from build123d import *

# Parameters (mm, degrees)
SKETCH1_W             = 9.495809557
SKETCH1_H             = 5.4
BOSS_EXTRUDE1_DEPTH   = 10
SKETCH1_H_2           = 5.02
BOSS_EXTRUDE1_2_DEPTH = 10
SKETCH1_H_3           = 4.94
BOSS_EXTRUDE1_3_DEPTH = 10
BOSS_EXTRUDE1_4_DEPTH = 10
BOSS_EXTRUDE1_5_DEPTH = 10
BOSS_EXTRUDE2_DEPTH   = 10
BOSS_EXTRUDE3_DEPTH   = 10
FILLET1_R             = 4
SKETCH6_R             = 2.5
CUT_EXTRUDE1_DEPTH    = 55


with BuildPart() as part:
    # Sketch1 → Boss-Extrude1 (new body)
    with BuildSketch(Plane.XY):
        with Locations((9.321382843, 6.543931341)):
            Rectangle(SKETCH1_W, SKETCH1_H)
    extrude(amount=-BOSS_EXTRUDE1_DEPTH)



with BuildPart() as body_2:
    # Sketch1 → Boss-Extrude1 2 (new body)
    with BuildSketch(Plane.XY):
        with Locations((9.321382843, 16.273802043)):
            Rectangle(SKETCH1_W, SKETCH1_H_2)
    extrude(amount=-BOSS_EXTRUDE1_2_DEPTH)


with BuildPart() as body_3:
    # Sketch1 → Boss-Extrude1 3 (new body)
    with BuildSketch(Plane.XY):
        with Locations((9.321382843, 26.315620999)):
            Rectangle(SKETCH1_W, SKETCH1_H_3)
    extrude(amount=-BOSS_EXTRUDE1_3_DEPTH)


with BuildPart() as body_4:
    # Sketch1 → Boss-Extrude1 4 (new body)
    with BuildSketch(Plane.XY):
        with Locations((9.321382843, 36.315620999)):
            Rectangle(SKETCH1_W, SKETCH1_H_3)
    extrude(amount=-BOSS_EXTRUDE1_4_DEPTH)


with BuildPart() as body_5:
    # Sketch1 → Boss-Extrude1 5 (new body)
    with BuildSketch(Plane.XY):
        Polygon((4.573645694, 48.785620997), (4.573479076, 43.845621), (14.069286609, 43.845621), (14.069119991, 48.785620997), align=None)
    extrude(amount=-BOSS_EXTRUDE1_5_DEPTH)


with BuildPart() as part_1:
    add(part.part)

    add(body_2.part)  # Boss-Extrude2 merges body 2

    add(body_3.part)  # Boss-Extrude2 merges body 3

    add(body_4.part)  # Boss-Extrude2 merges body 4

    add(body_5.part)  # Boss-Extrude2 merges body 5
    # Boss-Extrude2: read off the stored shape, not the designer's step
    # Boss-Extrude2 outline → Boss-Extrude2 (add)
    with BuildSketch(Plane.XY):
        Polygon((10.164012515, -23.151739204), (12.780095601, -3.151737932), (12.780095601, 48.785620997), (8.038968881, 48.785620997), (8.038703883, 51.848260515), (3.297312166, 51.848260515), (3.297312166, -3.151737932), (5.92637416, -23.151739204), align=None)
    extrude(amount=BOSS_EXTRUDE2_DEPTH)

    # Sketch3 → Boss-Extrude3 (add)
    with BuildSketch(Plane(origin=(0, 0, 0), x_dir=(-1, 0, 0), z_dir=(0, 0, -1))):
        Polygon((-4.573478064, -1.184377448), (-14.056261499, -1.184377448), (-10.164012515, -23.151739204), (-5.92637416, -23.151739204), align=None)
    extrude(amount=BOSS_EXTRUDE3_DEPTH)

    # Fillet1
    # the kernel refuses this fillet: 4 mm, written as the material it takes off along each edge
    with BuildSketch(Plane(origin=(15.800919998, 8.662254805, -10), x_dir=(0, 0, 1), z_dir=(-0.17446584987640118, -0.9846632252841095, 0))) as fillet1_piece_1:
        with BuildLine():
            CenterArc((FILLET1_R, FILLET1_R), FILLET1_R, 180, 90)
            Line((0, FILLET1_R), (0, 0))
            Line((0, 0), (FILLET1_R, 0))
        make_face()
    extrude(amount=42.309517805, mode=Mode.SUBTRACT)
    with BuildSketch(Plane(origin=(6.54107595, -33.132828409, -10), x_dir=(0, 0, 1), z_dir=(-0.06147017908550384, 0.9981089204506671, 0))) as fillet1_piece_2:
        with BuildLine():
            CenterArc((FILLET1_R, FILLET1_R), FILLET1_R, 180, 90)
            Line((0, FILLET1_R), (0, 0))
            Line((0, 0), (FILLET1_R, 0))
        make_face()
    extrude(amount=42.008982493, mode=Mode.SUBTRACT)
    with BuildSketch(Plane(origin=(4.573982978, 58.785620992, -10), x_dir=(0, 0, 1), z_dir=(-3.372835133255536e-05, -0.9999999994311992, 0))) as fillet1_piece_3_section:
        with BuildLine():
            CenterArc((FILLET1_R, -FILLET1_R), FILLET1_R, 90, 90)
            Line((0, -FILLET1_R), (0, 0))
            Line((0, 0), (FILLET1_R, 0))
        make_face()
    fillet1_piece_3 = extrude(amount=24.94, mode=Mode.PRIVATE)
    fillet1_piece_3 = split(fillet1_piece_3, bisect_by=Plane(origin=(4.573982978, 38.785620999, -10), z_dir=(0, 1, 0)), keep=Keep.TOP, mode=Mode.PRIVATE)
    add(fillet1_piece_3, mode=Mode.SUBTRACT)
    with BuildSketch(Plane(origin=(14.069623892, 33.845621006, -10), x_dir=(0, 0, 1), z_dir=(-3.372835144025149e-05, 0.9999999994311992, 0)), Plane(origin=(14.069287621, 23.845620999, -10), x_dir=(0, 0, 1), z_dir=(0, 1, 0)), Plane(origin=(14.069287621, 13.845620999, -10), x_dir=(0, 0, 1), z_dir=(0, 1, 0))) as fillet1_piece_4:
        with BuildLine():
            CenterArc((FILLET1_R, -FILLET1_R), FILLET1_R, 90, 90)
            Line((0, -FILLET1_R), (0, 0))
            Line((0, 0), (FILLET1_R, 0))
        make_face()
    extrude(amount=24.94, mode=Mode.SUBTRACT)
    with BuildSketch(Plane(origin=(14.069287621, 3.763802043, -10), x_dir=(0, 0, 1), z_dir=(0, 1, 0))) as fillet1_piece_5:
        with BuildLine():
            CenterArc((FILLET1_R, -FILLET1_R), FILLET1_R, 90, 90)
            Line((0, -FILLET1_R), (0, 0))
            Line((0, 0), (FILLET1_R, 0))
        make_face()
    extrude(amount=25.02, mode=Mode.SUBTRACT)
    with BuildSketch(Plane(origin=(14.069287621, -6.156068659, -10), x_dir=(-1, 0, 0), z_dir=(0, 1, 0))) as fillet1_piece_6:
        with BuildLine():
            CenterArc((FILLET1_R, FILLET1_R), FILLET1_R, 180, 90)
            Line((0, FILLET1_R), (0, 0))
            Line((0, 0), (FILLET1_R, 0))
        make_face()
    extrude(amount=25.4, mode=Mode.SUBTRACT)
    with BuildSketch(Plane(origin=(4.573478064, 19.243931341, -10), x_dir=(0, 0, 1), z_dir=(0, -1, 0))) as fillet1_piece_7_section:
        with BuildLine():
            CenterArc((FILLET1_R, -FILLET1_R), FILLET1_R, 90, 90)
            Line((0, -FILLET1_R), (0, 0))
            Line((0, 0), (FILLET1_R, 0))
        make_face()
    fillet1_piece_7 = extrude(amount=25.4, mode=Mode.PRIVATE)
    fillet1_piece_7 = split(fillet1_piece_7, bisect_by=Plane(origin=(4.573478064, 13.763802043, -10), z_dir=(0, -1, 0)), keep=Keep.TOP, mode=Mode.PRIVATE)
    add(fillet1_piece_7, mode=Mode.SUBTRACT)

    # Loft2: read off the stored shape, not the designer's step
    # Loft2: loft between two sections, ruled curve by curve
    loft2_from = [
        Edge.make_bspline([(12.780095601, -3.151737932, 10), (12.780095601, 5.504488557, 10), (12.780095601, 14.160715045, 10), (12.780095601, 31.473168021, 10), (12.780095601, 40.129394509, 10), (12.780095601, 48.785620997, 10)], [0, 0, 0, 0, 0.5, 0.5, 1, 1, 1, 1], 3),
        Edge.make_bspline([(4.573645694, 48.785620997, 10), (4.573617756, 40.457287923, 10), (4.573589817, 32.128954849, 10), (4.573533941, 15.472288701, 10), (4.573506003, 7.143955626, 10), (4.573478064, -1.184377448, 10)], [0, 0, 0, 0, 0.5, 0.5, 1, 1, 1, 1], 3),
        Edge.make_bspline([(4.573478064, -1.184377448, 10), (4.798960747, -4.845604407, 10), (5.024443429, -8.506831367, 10), (5.475408794, -15.829285285, 10), (5.700891477, -19.490512245, 10), (5.92637416, -23.151739204, 10)], [0, 0, 0, 0, 0.5, 0.5, 1, 1, 1, 1], 3),
        Edge.make_bspline([(10.164012515, -23.151739204, 10), (10.600026362, -19.818405659, 10), (11.03604021, -16.485072113, 10), (11.908067905, -9.818405022, 10), (12.344081753, -6.485071477, 10), (12.780095601, -3.151737932, 10)], [0, 0, 0, 0, 0.5, 0.5, 1, 1, 1, 1], 3),
        Edge.make_line((10.164012515, -23.151739204, 10), (5.92637416, -23.151739204, 10)),
        Edge.make_line((4.573645694, 48.785620997, 10), (12.780095601, 48.785620997, 10)),
    ]
    loft2_to = [
        Edge.make_bspline([(9.030825072, -23.151739204, 60), (9.427276266, -11.162179171, 60), (9.823727461, 0.827380863, 60), (10.616629851, 24.80650093, 60), (11.013081046, 36.796060964, 60), (11.409532241, 48.785620997, 60)], [0, 0, 0, 0, 0.5, 0.5, 1, 1, 1, 1], 3),
        Edge.make_bspline([(9.409532241, 48.785620997, 60), (9.13430376, 40.462103653, 60), (8.859075279, 32.138586309, 60), (8.308618317, 15.491551622, 60), (8.033389836, 7.168034278, 60), (7.758161355, -1.155483066, 60)], [0, 0, 0, 0, 0.5, 0.5, 1, 1, 1, 1], 3),
        Edge.make_bspline([(7.758161355, -1.155483066, 60), (7.636938641, -4.821525756, 60), (7.515715927, -8.487568446, 60), (7.273270499, -15.819653825, 60), (7.152047785, -19.485696515, 60), (7.030825072, -23.151739204, 60)], [0, 0, 0, 0, 0.5, 0.5, 1, 1, 1, 1], 3),
        Edge.make_bspline([(7.378058471, -23.151739204, 60), (7.653519571, -23.151739204, 60), (7.928980671, -23.151739204, 60), (8.479902871, -23.151739204, 60), (8.755363971, -23.151739204, 60), (9.030825072, -23.151739204, 60)], [0, 0, 0, 0, 0.5, 0.5, 1, 1, 1, 1], 3),
        Edge.make_line((7.378058471, -23.151739204, 60), (7.030825072, -23.151739204, 60)),
        Edge.make_line((9.409532241, 48.785620997, 60), (11.409532241, 48.785620997, 60)),
    ]
    loft2 = Solid(Shell([*[Face.make_surface_from_curves(loft2_from[k], loft2_to[k]) for k in range(6)], Face(Wire(loft2_from)), Face(Wire(loft2_to))]))
    add(loft2)

    # Sketch6 → Cut-Extrude1 (cut)
    with BuildSketch(Plane(origin=(0, 48.785620997, 0), x_dir=(1, 0, 0), z_dir=(0, 1, 0))):
        with Locations(Location((9.321382843, 5, 0), (0, 0, 270))):
            Circle(SKETCH6_R)
    extrude(amount=-CUT_EXTRUDE1_DEPTH, mode=Mode.SUBTRACT)


solid = part_1.part
Read the model definition and answer for the solid it produces. Units are mm, in the model's axes. A direction names the side the tool comes from. Round coordinates to 2 decimals unless told otherwise and drop trailing zeros. Write each loop counter-clockwise with the first axis right and the second up, starting at its lowest first coordinate (ties: lowest second). Pieces come first, ordered by that corner, then holes.
1. Given pin 1 Ø10 at (y, z) = (0.5, 23) entering from -X; pin 2 Ø4 at (x, z) = (9.32, -5) entering from +Y; pin 3 Ø5 at (y, z) = (33.5, 43.5) entering from +X, each flat-ended and moving along its own axis, determine where each tip first touches the part or whether it passes through.
2. The part is cut by section A-A, the plane z = -1.5. Determine the outline of the cut face in (x, y), then the cut area to 3 significant figures.
3. Straight lines are drawn through the part: L1, parallel to Y at x = 8, z = -2; L2, parallel to X at y = 6, z = -5; L3, parallel to Z at x = 9.5, y = 6. For each, find the intervals that lie inside material, in ascending order.
4. Determine the mould class of faces 1 (the face through (7, 33.846, -3)), 2 (the face through (14.069, 26, -3)), 3 (the face through (6.01, -12.34, -8.33)), 4 (the face through (7, 32, 0)) for opening direction Y: pulls with the +Y half, pulls with the -Y half, needs draft (parallel to the pull), parting line crosses it, or undercut.
5. Which of the six approach directions +Z, -Z, +X, -X, +Y, -Y give full straight-line access (tool end or side, diameter ignored) to faces 5 (the face through (12.6, -8, 0)), 6 (the face through (7, 3.844, -3)), 7 (the face through (5.714, 46.35, -8.797))?
Values:
1. pin 1: stops at x = 5.09
1. pin 2: stops at y = -6.21
1. pin 3: stops at x = 11.6
2. outline: (4.57, -1.18) - (5.93, -23.15) - (10.16, -23.15) - (14.06, -1.18) - close; (4.57, 3.84) - (14.07, 3.84) - (14.07, 9.24) - (4.57, 9.24) - close; (4.57, 13.76) - (14.07, 13.76) - (14.07, 18.78) - (4.57, 18.78) - close; (4.57, 23.85) - (14.07, 23.85) - (14.07, 28.79) - (4.57, 28.79) - close; (4.57, 33.85) - (14.07, 33.85) - (14.07, 38.79) - (4.57, 38.79) - close; (4.57, 43.85) - (14.07, 43.85) - (14.07, 48.79) - (4.57, 48.79) - close
2. area: 390 mm2
3. L1: y = -23.15 to -1.18, 3.84 to 9.24, 13.76 to 18.78, 23.85 to 28.79, 33.85 to 38.79, 43.85 to 48.79
3. L2: x = 4.57 to 6.82, 11.82 to 14.07
3. L3: z = -10 to -7.49, -2.51 to 60
4. face 1: undercut
4. face 2: needs draft
4. face 3: pulls with the -Y half
4. face 4: undercut
5. face 5: +Z, +X, -Y
5. face 6: -Z, +X, -X
5. face 7: -Z, -X, +Y
